The model under review builds one solid part; all positions refer to its coordinate system, in mm. Round coordinates to 2 decimals unless told otherwise and drop trailing zeros. Write each loop counter-clockwise with the first axis right and the second up, starting at its lowest first coordinate (ties: lowest second). Pieces come first, ordered by that corner, then holes. Notation, with made-up numbers: (28, -37) - (64, -37) arc R33 cw to (64, -5) - close; hole circle Ø9 at (-35.75, 45.25). An arc over 180 degrees is marked (long way). Return JSON: item names as keys, results as strings.
from build123d import *

# Parameters (mm, degrees)
F1_DEPTH = 38.1
F3_DEPTH = 6.35


with BuildPart() as f1:
    # F0 (on Front) → F1 (new body)
    with BuildSketch(Plane.XZ):
        Polygon((21.9970452561, -38.1), (-21.9970452561, -38.1), (0, -76.2), (424.2044321158, -810.9436292205), (457.2, -791.8936292205), align=None)
        Polygon((65.9911357684, -38.1), (21.9970452561, -38.1), (457.2, -791.8936292205), (490.1955678842, -772.8436292205), align=None)
        Polygon((914.4, 0), (0, 0), (21.9970452561, -38.1), (65.9911357684, -38.1), (914.4, -38.1), align=None)
        Polygon((21.9970452561, 38.1), (0, 0), (914.4, 0), (914.4, 38.1), (65.9911357684, 38.1), align=None)
        Polygon((457.2, 791.8936292205), (21.9970452561, 38.1), (65.9911357684, 38.1), (490.1955678842, 772.8436292205), align=None)
        Polygon((0, 76.2), (21.9970452561, 38.1), (457.2, 791.8936292205), (424.2044321158, 810.9436292205), align=None)
        Polygon((-21.9970452561, 38.1), (21.9970452561, 38.1), (0, 76.2), (-424.2044321158, 810.9436292205), (-457.2, 791.8936292205), align=None)
        Polygon((-65.9911357684, 38.1), (-21.9970452561, 38.1), (-457.2, 791.8936292205), (-490.1955678842, 772.8436292205), align=None)
        Polygon((-21.9970452561, -38.1), (0, 0), (-914.4, 0), (-914.4, -38.1), (-65.9911357684, -38.1), align=None)
        Polygon((-914.4, 0), (0, 0), (-21.9970452561, 38.1), (-65.9911357684, 38.1), (-914.4, 38.1), align=None)
        Polygon((-457.2, -791.8936292205), (-21.9970452561, -38.1), (-65.9911357684, -38.1), (-490.1955678842, -772.8436292205), align=None)
        Polygon((0, -76.2), (-21.9970452561, -38.1), (-457.2, -791.8936292205), (-424.2044321158, -810.9436292205), align=None)
        Polygon((-21.9970452561, 38.1), (0, 0), (21.9970452561, 38.1), align=None)
        Polygon((21.9970452561, -38.1), (0, 0), (-21.9970452561, -38.1), align=None)
    extrude(amount=-F1_DEPTH)

    # F2 (on face) → F3 (join)
    with BuildSketch(Plane.XZ):
        with BuildLine():
            ThreePointArc((65.9911357684, -38.1), (73.6035479632, -19.7220112368), (76.2, 0))
            ThreePointArc((76.2, 0), (73.6035479632, 19.7220112368), (65.9911357684, 38.1))
            ThreePointArc((65.9911357684, 38.1), (38.1, 65.9911357684), (0, 76.2))
            ThreePointArc((0, 76.2), (-38.1, 65.9911357684), (-65.9911357684, 38.1))
            ThreePointArc((-65.9911357684, 38.1), (-76.2, 0), (-65.9911357684, -38.1))
            ThreePointArc((-65.9911357684, -38.1), (-38.1, -65.9911357684), (0, -76.2))
            ThreePointArc((0, -76.2), (38.1, -65.9911357684), (65.9911357684, -38.1))
        make_face()
    extrude(amount=F3_DEPTH)


solid = f1.part
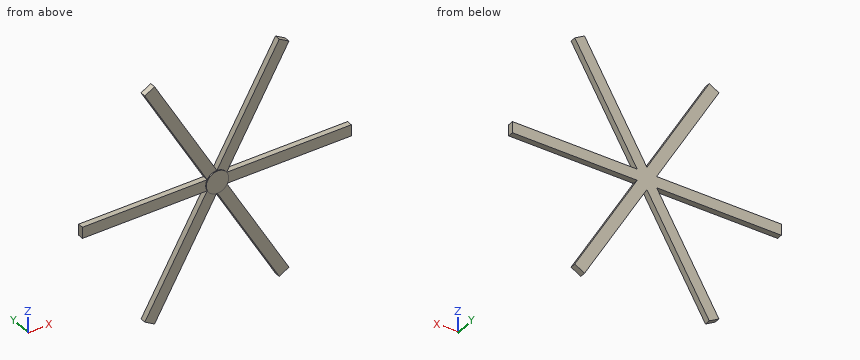
(1) Clearance check with flat-ended pins moving along their axes: pin 1 Ø19 at (x, y) = (335.5, 22) entering from +Z; pin 2 Ø10 at (x, y) = (600.5, 12) entering from -Z; pin 3 Ø23 at (x, z) = (438.5, 5) entering from -Y. State where each tip first meets the part, or that it passes through.
Filled in:
{"pin 1": "stops at z = 673.76", "pin 2": "stops at z = -38.1", "pin 3": "stops at y = 0"}
(2) Add section C-C (z = 640). Write out the cut boundary in (x, y), plus the area to 3 significant figures.
Filled in:
{"outline": "(-413.5, 0) - (-325.51, 0) - (-325.51, 38.1) - (-413.5, 38.1) - close; (325.51, 0) - (413.5, 0) - (413.5, 38.1) - (325.51, 38.1) - close", "area": "6,700 mm2"}
(3) Add section A-A (x = -392). Write out the cut boundary in (y, z).
Filled in:
{"outline": "(0, -755.16) - (38.1, -755.16) - (38.1, -602.76) - (0, -602.76) - close; (0, -38.1) - (38.1, -38.1) - (38.1, 38.1) - (0, 38.1) - close; (0, 602.76) - (38.1, 602.76) - (38.1, 755.16) - (0, 755.16) - close"}
(4) Add section B-B (y = 16). Write out the cut boundary in (x, z), plus the area to 3 significant figures.
Filled in:
{"outline": "(-914.4, -38.1) - (-65.99, -38.1) - (-490.2, -772.84) - (-424.2, -810.94) - (0, -76.2) - (424.2, -810.94) - (490.2, -772.84) - (65.99, -38.1) - (914.4, -38.1) - (914.4, 38.1) - (65.99, 38.1) - (490.2, 772.84) - (424.2, 810.94) - (0, 76.2) - (-424.2, 810.94) - (-490.2, 772.84) - (-65.99, 38.1) - (-914.4, 38.1) - close", "area": "403,000 mm2"}
(5) Add section D-D (x = 652). Write out the cut boundary in (y, z).
Filled in:
{"outline": "(0, -38.1) - (38.1, -38.1) - (38.1, 38.1) - (0, 38.1) - close"}
(6) Wall thickness on line 1 (Z direction, x = -122.5, y = 2.5); line 2 (Z direction, x = 349.5, y = 32); line 3 (Z direction, x = -522.5, y = 13): over which ranges is each line inside the solid? List them lowest first.
Filled in:
{"line 1": "z = -288.38 to -135.98, -38.1 to 38.1, 135.98 to 288.38", "line 2": "z = -681.55 to -529.15, -38.1 to 38.1, 529.15 to 681.55", "line 3": "z = -38.1 to 38.1"}
